Input: dimensioned drawing with shaded views. Units: mm. Origin: part minimum x, y, z. Round coordinates to 2 decimals unless told otherwise and drop trailing zeros. Loops run counter-clockwise (first coordinate to the right, second up) from the corner with the lowest first, then second, coordinate; pieces in that order, holes last. Notation, with made-up numbers: (-7, 38) - (26, 38) arc R15 ccw to (26, 67) - close; hole circle Ø11 at (6, -28.75). An arc over 180 degrees is marked (long way). One line per question, with ' | ' between items. Start each with the question number.
Item 1: Section A-A, the plane y = 5. Return loops of the section in (x, z).
Item 2: Section B-B, the plane x = 58.5. Return loops of the section in (y, z), plus the area to 3 significant figures.
Item 3: Draft query along X for the marked faces 1, 2, 3 and 4. Return one class per face: pulls with the +X half, pulls with the -X half, needs draft (parallel to the pull), parting line crosses it, or undercut.
Item 4: Material intervals for line 1 along X through (y, z) = (29.5, 1.5); line 2 along Y through (x, z) = (127.95, 7.5); line 3 along Y through (x, z) = (50, 9.5), sorted ascending.
Item 5: First-contact query: pin 1 (4 mm diameter, centred on x = 71.5, z = 7, fed in from +Y). Flat tip, straight axial feed; report the tip coordinate or a pass-through.
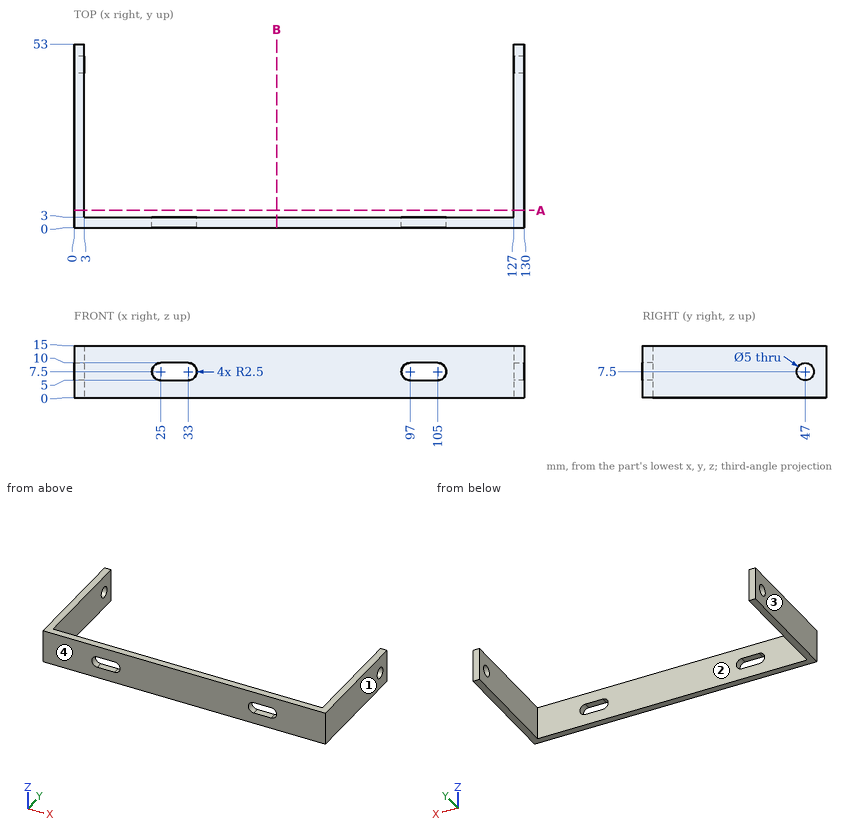
Return value:
1) outline: (0, 0) - (3, 0) - (3, 15) - (0, 15) - close; (127, 0) - (130, 0) - (130, 15) - (127, 15) - close
2) outline: (0, 0) - (3, 0) - (3, 15) - (0, 15) - close | area: 45.0 mm2
3) face 1: pulls with the +X half | face 2: undercut | face 3: pulls with the -X half | face 4: needs draft
4) line 1: 0 to 3, 127 to 130 | line 2: 0 to 44.5, 49.5 to 53 | line 3: 0 to 3
5) pin 1: y = 3
